from build123d import *

# Parameters (mm, degrees)
SKETCH1_W           = 150
SKETCH1_H           = 150
BOSS_EXTRUDE1_DEPTH = 5
FILLET1_R           = 10
SKETCH2_R           = 2
CUT_EXTRUDE1_DEPTH  = 107.183802908


with BuildPart() as part:
    # Sketch1 → Boss-Extrude1 (new body)
    with BuildSketch(Plane(origin=(0, 0, 0), x_dir=(1, 0, 0), z_dir=(0, 1, 0))):
        Rectangle(SKETCH1_W, SKETCH1_H)
    extrude(amount=BOSS_EXTRUDE1_DEPTH)

    # Fillet1
    fillet1_edges = [part.edges().sort_by_distance(p)[0] for p in [
        (-75, 2.5, -75),
        (-75, 2.5, 75),
        (75, 2.5, 75),
        (75, 2.5, -75),
    ]]
    fillet(fillet1_edges, radius=FILLET1_R)

    # Sketch2 → Cut-Extrude1 (cut, through all)
    with BuildSketch(Plane(origin=(0, 5, 0), x_dir=(1, 0, 0), z_dir=(0, 1, 0))):
        with Locations(Location((65, 65, 0), (0, 0, 270))):
            Circle(SKETCH2_R)
        with Locations(Location((-65, 65, 0), (0, 0, 270))):
            Circle(SKETCH2_R)
        with Locations(Location((-65, -65, 0), (0, 0, 270))):
            Circle(SKETCH2_R)
        with Locations(Location((65, -65, 0), (0, 0, 270))):
            Circle(SKETCH2_R)
    extrude(amount=-CUT_EXTRUDE1_DEPTH, mode=Mode.SUBTRACT)


solid = part.part
Geometry: final body of the model. Coordinates: model frame, mm. Give positions to 0.01 mm unless a question says otherwise; leave off trailing zeros. Answer in a Markdown table with one row per item. Add a question column.
(1) Mould query, pull axis Z, two halves, no side actions, for faces 1 (the cylindrical face through (67, 3, -65)), 2 (the flat face through (-1, 2, -75)), 3 (the flat face through (-1, 5, -1)). Classes: +Z half, -Z half, draft (parallel to the pull), parting line (faces both ways), or undercut.
(2) Ray query, line 1 (X direction, y = 3, z = -65); line 2 (Z direction, x = -66.5, y = 2.05). Return the intervals inside material, ascending.
(3) First-contact query: pin 1 (5 mm diameter, centred on x = 65, z = -65, fed in from +Y). Flat tip, straight axial feed; report the tip coordinate or a pass-through.
Result set:
| question | item | result |
|---|---|---|
| 1 | face 1 | undercut |
| 1 | face 2 | -Z half |
| 1 | face 3 | draft |
| 2 | line 1 | x = -75 to -67, -63 to 63, 67 to 75 |
| 2 | line 2 | z = -74.89 to -66.32, -63.68 to 63.68, 66.32 to 74.89 |
| 3 | pin 1 | stops at y = 5 |
